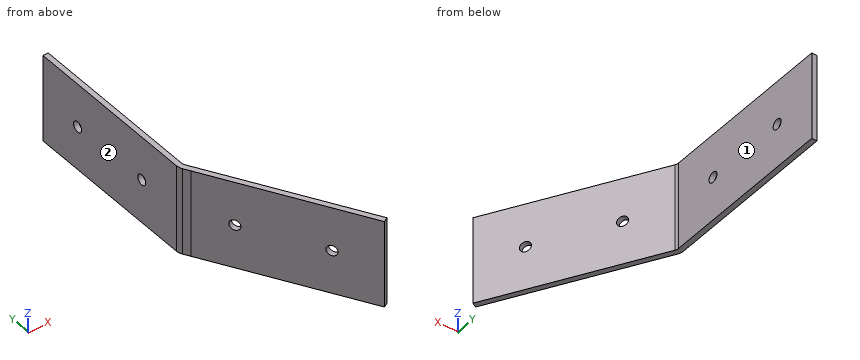
from build123d import *

# Parameters (mm, degrees)
SKETCH1_W                = 101.6
SKETCH1_H                = 25.4
BASE_FLANGE1_DEPTH       = 1.51892
SKETCHED_START           = -12.7
SKETCHED_BEND1_DEPTH     = 25.4
SKETCHED_BEND1_2_DEPTH   = 25.4
F_3_0_3_DIAMETER_HOLE1_D = 3
F_3_0_3_DIAMETER_HOLE2_D = 3


# Read off the part's stored shape, not the designer's step: Sketched Bend1
# Sheet-metal steps are written as plain solids
with BuildPart() as part:
    # Sketch1 → Base-Flange1 (new body)
    with BuildSketch(Plane.YZ):
        Rectangle(SKETCH1_W, SKETCH1_H)
    extrude(amount=-BASE_FLANGE1_DEPTH)

    # Sketched Bend1 outline → Sketched Bend1 (cut)
    with BuildSketch(Plane.XY.offset(SKETCHED_START)):
        with BuildLine():
            Line((0, -2.850729215), (-1.060201701, -1.014406003))
            ThreePointArc((-1.060201701, -1.014406003), (-1.402252755, -0.188621708), (-1.51892, 0.697553997))
            Line((-1.51892, 0.697553997), (-1.51892, -50.8))
            Line((-1.51892, -50.8), (0, -50.8))
            Line((0, -50.8), (0, -2.850729215))
        make_face()
    extrude(amount=SKETCHED_BEND1_DEPTH, mode=Mode.SUBTRACT)

    # Sketched Bend1 2 outline → Sketched Bend1 2 (add)
    with BuildSketch(Plane.XY.offset(SKETCHED_START)):
        with BuildLine():
            Line((0, 0.697553997), (0, -2.850729215))
            Line((0, -2.850729215), (23.991021301, -44.404397034))
            Line((23.991021301, -44.404397034), (25.306444607, -43.644937034))
            Line((25.306444607, -43.644937034), (0.255221606, -0.254946003))
            ThreePointArc((0.255221606, -0.254946003), (0.064911301, 0.204503716), (0, 0.697553997))
        make_face()
    extrude(amount=SKETCHED_BEND1_2_DEPTH)

    # Ø3.0 (3) Diameter Hole1 (through all)
    with Locations(Plane(origin=(0.081021347, 0.046777696, 0), x_dir=(-0.500000000000001, 0.866025403784438, 0), z_dir=(0.866025403784438, 0.500000000000001, 0))):
        with Locations((-37.450846521, 0), (-13.348400518, 0)):
            Hole(F_3_0_3_DIAMETER_HOLE1_D / 2)

    # Ø3.0 (3) Diameter Hole2 (through all)
    with Locations(Plane.YZ):
        with Locations((13.697553997, 0), (37.8, 0)):
            Hole(F_3_0_3_DIAMETER_HOLE2_D / 2)


solid = part.part
Input: part model. Units: mm. Frame: model coordinates. Face numbers are marked on the shaded views. A direction names the side the tool comes from. Coordinates: 2 decimals unless noted, no trailing zeros. Write each loop counter-clockwise with the first axis right and the second up, starting at its lowest first coordinate (ties: lowest second). Pieces come first, ordered by that corner, then holes. Notation, with made-up numbers: M 35,-30.75 L 58,-30.75 A25 ccw 58,-11.75 Z; hole C -7,-36 d9. An arc over 180 degrees is marked long. Answer as a JSON object with one key per item and string values. Group by question number.
(1) Section A-A on y = 37.8. Output: boundary loops of the cut face in (x, z), plus the area to 3 significant figures.
(2) Section B-B on z = 0. Output: boundary loops of the cut face in (x, y) (3 decimals), plus the area to 3 significant figures.
(3) Set-up query: the marked faces 1 and 2. Return all of +Z, -Z, +X, -X, +Y, -Y with unobstructed straight access to the full face (end or side cutting, diameter ignored); none if empty.
(4) Ray query, line 1 along Z through (x, y) = (-0.25, 37.8); line 2 along X through (y, z) = (35, 4.5); line 3 along Y through (x, z) = (11, 3.25). Return the intervals inside material, ascending. Write a range as [from, to].
(5) Contact query for flat-ended pins moving along their axis: P1, Ø5, axis at x = 11.5, z = -9.5, coming from the +Y side; P2, Ø1.5, axis at x = 20, z = -0.5, coming from the +Y side; P3, Ø3.5, axis at y = 13.7, z = 0, coming from the -X side; P4, Ø6, axis at x = 7.5, z = -3, coming from the -Y side. Output: stop coordinate, or through.
(6) Section C-C on z = 8.75. Output: boundary loops of the cut face in (x, y) (3 decimals), plus the area to 3 significant figures.
(7) Section D-D on y = 26.5. Output: boundary loops of the cut face in (x, z), plus the area to 3 significant figures.
Result set:
{
 "1": {"outline": "M -1.52,-12.7 L 0,-12.7 L 0,-1.5 L -1.52,-1.5 Z; M -1.52,1.5 L 0,1.5 L 0,12.7 L -1.52,12.7 Z", "area": "34.0 mm2"},
 "2": {"outline": "M -1.519,0.698 A3.424 ccw -1.06,-1.014 L 4.69,-10.974 L 6.005,-10.214 L 0.255,-0.255 A1.905 cw 0,0.698 L 0,12.198 L -1.519,12.198 Z; M -1.519,15.198 L 0,15.198 L 0,36.3 L -1.519,36.3 Z; M -1.519,39.3 L 0,39.3 L 0,50.8 L -1.519,50.8 Z; M 6.19,-13.572 L 16.741,-31.847 L 18.056,-31.088 L 7.505,-12.812 Z; M 18.241,-34.445 L 23.991,-44.404 L 25.306,-43.645 L 19.556,-33.686 Z", "area": "136 mm2"},
 "3": {"face 1": "+Z, -Z, +X, +Y", "face 2": "+Z, -Z, -X, +Y, -Y"},
 "4": {"line 1": "z = [-12.7, -1.5], [1.5, 12.7]", "line 2": "x = [-1.52, 0]", "line 3": "y = [-21.9, -18.87]"},
 "5": {"P1": "stops at y = -15.4", "P2": "stops at y = -33.4", "P3": "stops at x = -1.52", "P4": "stops at y = -21.04"},
 "6": {"outline": "M -1.519,0.698 A3.424 ccw -1.06,-1.014 L 23.991,-44.404 L 25.306,-43.645 L 0.255,-0.255 A1.905 cw 0,0.698 L 0,50.8 L -1.519,50.8 Z", "area": "154 mm2"},
 "7": {"outline": "M -1.52,-12.7 L 0,-12.7 L 0,12.7 L -1.52,12.7 Z", "area": "38.6 mm2"}
}
